```python
from build123d import *

# Parameters (mm, degrees)
SKETCH005_W            = 50
SKETCH005_H            = 70
PAD003_DEPTH           = 3
SKETCH006_W            = 10
SKETCH006_H            = 3
POCKET002_DEPTH        = 5
LINEARPATTERN003_COUNT = 9
LINEARPATTERN003_PITCH = 10


with BuildPart() as part:
    # Sketch005 → Pad003 (new body)
    with BuildSketch(Plane.XZ):
        Polygon((-40, 50), (-30, 50), (-25, 45), (25, 45), (30, 50), (40, 50), (40, -50), (30, -50), (25, -45), (-25, -45), (-30, -50), (-40, -50), align=None)
        Rectangle(SKETCH005_W, SKETCH005_H, mode=Mode.SUBTRACT)
    extrude(amount=PAD003_DEPTH)

    # Sketch006 → Pocket002 (cut)
    with BuildSketch(Plane(origin=(0, 0, -40), x_dir=(1, 0, 0), z_dir=(0, -1, 0))):
        with Locations((-37.5, 0)):
            Rectangle(SKETCH006_W, SKETCH006_H)
        with Locations((37.5, 0)):
            Rectangle(SKETCH006_W, SKETCH006_H)
    pocket002 = extrude(amount=POCKET002_DEPTH, mode=Mode.SUBTRACT)

    # LinearPattern003: Pocket002 ×9
    with Locations(*[(0, 0, i * LINEARPATTERN003_PITCH) for i in range(1, LINEARPATTERN003_COUNT)]):
        add(pocket002, mode=Mode.SUBTRACT)


with BuildPart() as part_1:
    # Body002 placement: moved
    add(part.part.moved(Location((0, 11.5, 10))))


with BuildPart() as part_2:
    # Body003 placement: moved
    add(part_1.part.moved(Location((0, 200, 0))))


solid = part_2.part
```
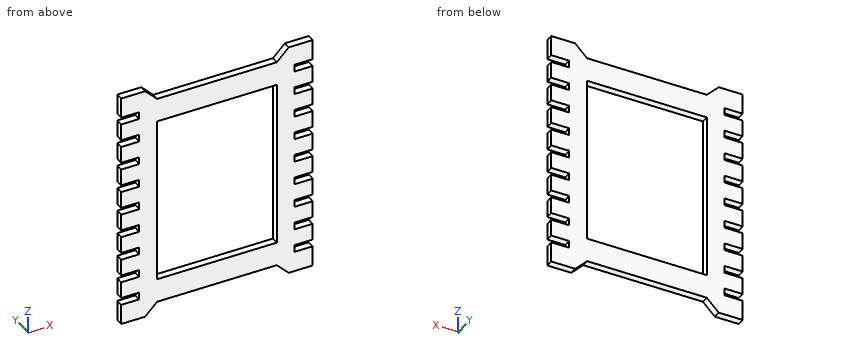
Geometry: final body of the model. Coordinates: model frame, mm. Round coordinates to 2 decimals unless told otherwise and drop trailing zeros. Order: outer loops, then holes, each group sorted by start corner. A loop starts at its lowest first (then second) coordinate and runs counter-clockwise, first axis right, second up. Notation, with made-up numbers: (71, -30.5) - (83, -30.5) arc R23 ccw to (83, -2.5) - close; hole circle Ø10 at (12.5, 32.5). An arc over 180 degrees is marked (long way). Write item = value, one per line. Start each with the question number.
Q1. Cut plane B-B on z = 5. Return the cut outline in (x, y), and give its area (3 significant figures).
Q2. Pin query (flat end, axial travel): pin 1 (1.5 mm diameter, centred on y = 210, z = 10, fed in from +X); pin 2 (0.9 mm diameter, centred on x = -12, y = 209.5, fed in from -Z); pin 3 (0.9 mm diameter, centred on y = 210.5, z = 30.5, fed in from -X). Return the tip coordinate at first contact, or that it passes through.
Q3. Cut plane C-C on x = -27.5. Return the cut outline in (y, z), and give its area (3 significant figures).
Q4. Ray query, line 1 (X direction, y = 210.3, z = 43); line 2 (X direction, y = 209, z = 39); line 3 (Z direction, x = -10, y = 209.45). Return the intervals inside material, ascending. Write a range as from..to.
Q5. Cut plane A-A on x = -17.5. Return the cut outline in (y, z).
Outcome:
q1.outline = (-40, 208.5) - (-25, 208.5) - (-25, 211.5) - (-40, 211.5) - close; (25, 208.5) - (40, 208.5) - (40, 211.5) - (25, 211.5) - close
q1.area = 90.0 mm^2
q2.pin_1 = 32.5
q2.pin_2 = -35
q2.pin_3 = -32.5
q3.outline = (208.5, -37.5) - (211.5, -37.5) - (211.5, 57.5) - (208.5, 57.5) - close
q3.area = 285 mm^2
q4.line_1 = -40..-25, 25..40
q4.line_2 = -32.5..-25, 25..32.5
q4.line_3 = -35..-25, 45..55
q5.outline = (208.5, -35) - (211.5, -35) - (211.5, -25) - (208.5, -25) - close; (208.5, 45) - (211.5, 45) - (211.5, 55) - (208.5, 55) - close
